Input: part model. Units: mm. Frame: model coordinates. A direction names the side the tool comes from. Round coordinates to 2 decimals unless told otherwise and drop trailing zeros. Order: outer loops, then holes, each group sorted by start corner. A loop starts at its lowest first (then second) coordinate and runs counter-clockwise, first axis right, second up.
Item 1: Cut plane A-A on x = -31.5. Output: boundary loops of the cut face in (y, z).
Item 2: Mould query, pull axis Y, two halves, no side actions, for faces 4 (the flat face through (2, -25.4, 3)), 5 (the flat face through (47.625, 0, 3)), 6 (the cylindrical face through (-64.765, 23.589, 3.131)). Classes: released by +Y, released by -Y, zero draft, split by the parting line, or undercut.
Item 3: Reachability of faces 1 (the flat face through (-32, -9.652, 3)), 2 (the flat face through (26, -11.43, 3)), 3 (the flat face through (12, 0, 0)) from +Z, -Z, +X, -X, +Y, -Y: full face, straight path, thin tool, end or side. Return the list, or none.
Item 4: First-contact query: pin 1 (1.5 mm diameter, centred on y = 0, z = 4.5, fed in from +X) (3 decimals); pin 2 (1.9 mm diameter, centred on x = 77, z = 4.5, fed in from -Y); pin 3 (1.9 mm diameter, centred on y = -14.5, z = 2.5, fed in from +X); pin 4 (2 mm diameter, centred on x = -40.5, y = 8, fed in from -Z). Flat tips, straight axial feed; report the tip coordinate or a pass-through.
Item 5: Line query: L1, parallel to Y at x = 16, z = 1.75; L2, parallel to X at y = -16, z = 3.25 (3 decimals); L3, parallel to X at y = 11.5, z = 4.5 (3 decimals). Output: solid intervals per line, ascending.
Item 6: Cut plane C-C on z = 2.75. Give the number of separate pieces and of enclosed holes in the cut face, then the cut area to 3 significant figures.
Item 7: Cut plane B-B on x = 38.5. Output: boundary loops of the cut face in (y, z).
```python
from build123d import *

# Parameters (mm, degrees)
F0_R        = 3.175
F0_W        = 30.48
F0_H        = 5.08
F0_W_2      = 12.7
F0_W_3      = 71.12
F0_H_2      = 19.304
F1_DEPTH    = 6.35
F1_FACE_W   = 5.08
F1_FACE_H   = 12.7
F1_FACE_R   = 2.6543
F1_FACE_R_2 = 3.175
F1_FACE_W_2 = 30.48
F1_FACE_H_2 = 5.08
F1_FACE_W_3 = 12.7
F2_DEPTH    = 6.35
F3_DEPTH    = 93.98


with BuildPart() as f1:
    # F0 (on Top) → F1 (new body)
    with BuildSketch(Plane.XY):
        with BuildLine():
            Line((66.675, 19.05), (66.675, 25.4))
            Line((66.675, 25.4), (-60.325, 25.4))
            ThreePointArc((-60.325, 25.4), (-64.815128, 23.540128), (-66.675, 19.05))
            Line((-66.675, 19.05), (-66.675, 9.652))
            Line((-66.675, 9.652), (4.445, 9.652))
            Line((4.445, 9.652), (4.445, -9.652))
            Line((4.445, -9.652), (-66.675, -9.652))
            Line((-66.675, -9.652), (-66.675, -19.05))
            ThreePointArc((-66.675, -19.05), (-64.815128, -23.540128), (-60.325, -25.4))
            Line((-60.325, -25.4), (66.675, -25.4))
            Line((66.675, -25.4), (66.675, -19.05))
            Line((66.675, -19.05), (64.135, -19.05))
            Line((64.135, -19.05), (64.135, -6.35))
            Line((64.135, -6.35), (66.675, -6.35))
            Line((66.675, -6.35), (66.675, -2.6543))
            ThreePointArc((66.675, -2.6543), (64.0207, 0), (66.675, 2.6543))
            Line((66.675, 2.6543), (66.675, 6.35))
            Line((66.675, 6.35), (64.135, 6.35))
            Line((64.135, 6.35), (64.135, 19.05))
            Line((64.135, 19.05), (66.675, 19.05))
        make_face()
        with Locations((-47.448933, -17.526)):
            Circle(F0_R, mode=Mode.SUBTRACT)
        with Locations((26.035, -13.97)):
            Rectangle(F0_W, F0_H, mode=Mode.SUBTRACT)
        with Locations((53.975, 0)):
            Rectangle(F0_W_2, F0_H, mode=Mode.SUBTRACT)
        with Locations((-47.625, 17.526)):
            Circle(F0_R, mode=Mode.SUBTRACT)
        with Locations((26.035, 13.97)):
            Rectangle(F0_W, F0_H, mode=Mode.SUBTRACT)
        with BuildLine():
            ThreePointArc((66.675, -25.4), (92.075, 0), (66.675, 25.4))
            Line((66.675, 25.4), (66.675, 19.05))
            Line((66.675, 19.05), (69.215, 19.05))
            Line((69.215, 19.05), (69.215, 6.35))
            Line((69.215, 6.35), (66.675, 6.35))
            Line((66.675, 6.35), (66.675, 2.6543))
            ThreePointArc((66.675, 2.6543), (68.551874, 1.876874), (69.3293, 0))
            ThreePointArc((69.3293, 0), (68.551874, -1.876874), (66.675, -2.6543))
            Line((66.675, -2.6543), (66.675, -6.35))
            Line((66.675, -6.35), (69.215, -6.35))
            Line((69.215, -6.35), (69.215, -19.05))
            Line((69.215, -19.05), (66.675, -19.05))
            Line((66.675, -19.05), (66.675, -25.4))
        make_face()
        with Locations((79.375, 0)):
            Rectangle(F0_W_2, F0_H, mode=Mode.SUBTRACT)
        with Locations((-31.115, 0)):
            Rectangle(F0_W_3, F0_H_2)
    extrude(amount=F1_DEPTH)

    # F1_face (on face) → F2 (join)
    with BuildSketch(Plane(origin=(7.852921, 0, 6.35), x_dir=(1, 0, 0), z_dir=(0, 0, 1))):
        with BuildLine():
            Line((58.822079, 25.4), (-68.177921, 25.4))
            ThreePointArc((-68.177921, 25.4), (-72.668049, 23.540128), (-74.527921, 19.05))
            Line((-74.527921, 19.05), (-74.527921, -19.05))
            ThreePointArc((-74.527921, -19.05), (-72.668049, -23.540128), (-68.177921, -25.4))
            Line((-68.177921, -25.4), (58.822079, -25.4))
            ThreePointArc((58.822079, -25.4), (84.222079, 0), (58.822079, 25.4))
        make_face()
        with Locations((58.822079, 12.7)):
            Rectangle(F1_FACE_W, F1_FACE_H, mode=Mode.SUBTRACT)
        with Locations((58.822079, -12.7)):
            Rectangle(F1_FACE_W, F1_FACE_H, mode=Mode.SUBTRACT)
        with Locations((58.822079, 0)):
            Circle(F1_FACE_R, mode=Mode.SUBTRACT)
        with Locations((-55.301854, -17.526)):
            Circle(F1_FACE_R_2, mode=Mode.SUBTRACT)
        with Locations((18.182079, -13.97)):
            Rectangle(F1_FACE_W_2, F1_FACE_H_2, mode=Mode.SUBTRACT)
        with Locations((46.122079, 0)):
            Rectangle(F1_FACE_W_3, F1_FACE_H_2, mode=Mode.SUBTRACT)
        with Locations((-55.477921, 17.526)):
            Circle(F1_FACE_R_2, mode=Mode.SUBTRACT)
        with Locations((18.182079, 13.97)):
            Rectangle(F1_FACE_W_2, F1_FACE_H_2, mode=Mode.SUBTRACT)
        with Locations((71.522079, 0)):
            Rectangle(F1_FACE_W_3, F1_FACE_H_2, mode=Mode.SUBTRACT)
    extrude(amount=-F2_DEPTH)

    # F0 (on Top) → F3 (cut)
    with BuildSketch(Plane.XY):
        with Locations((-31.115, 0)):
            Rectangle(F0_W_3, F0_H_2)
    extrude(amount=F3_DEPTH, mode=Mode.SUBTRACT)


solid = f1.part
```
From the geometry:
1. outline: (-25.4, 0) - (-9.65, 0) - (-9.65, 6.35) - (-25.4, 6.35) - close; (9.65, 0) - (25.4, 0) - (25.4, 6.35) - (9.65, 6.35) - close
2. face 4: released by -Y
2. face 5: undercut
2. face 6: released by +Y
3. face 1: +Z, -Z, -X
3. face 2: +Z, -Z
3. face 3: -Z, +X, -X, +Y, -Y
4. pin 1: stops at x = 92.075
4. pin 2: stops at y = -23.61
4. pin 3: stops at x = 88.16
4. pin 4: passes through
5. L1: y = -25.4 to -16.51, -11.43 to 11.43, 16.51 to 25.4
5. L2: x = -66.675 to -50.233, -44.665 to 10.795, 41.275 to 64.135, 69.215 to 86.402
5. L3: x = -66.675 to 10.795, 41.275 to 64.135, 69.215 to 89.323
6. separate pieces: 1
6. enclosed holes: 9
6. area: 5,740 mm2
7. outline: (-25.4, 0) - (-16.51, 0) - (-16.51, 6.35) - (-25.4, 6.35) - close; (-11.43, 0) - (11.43, 0) - (11.43, 6.35) - (-11.43, 6.35) - close; (16.51, 0) - (25.4, 0) - (25.4, 6.35) - (16.51, 6.35) - close
